For this review, take the finished solid that the model builds, in its own axes (mm). Face numbers are marked on the shaded views. A direction names the side the tool comes from. Coordinates: 2 decimals unless noted, no trailing zeros. Order: outer loops, then holes, each group sorted by start corner. A loop starts at its lowest first (then second) coordinate and runs counter-clockwise, first axis right, second up. Notation, with made-up numbers: (3.25, 55) -> (47.25, 55) arc R35 cw to (47.25, 91) -> close; hole circle Ø5 at (-24.75, -2.5). An arc over 180 degrees is marked (long way). Answer as a JSON object with one key per item and string values. Group by question number.
1) Draft analysis for pull direction Y (two halves, no side actions). For the marked faces 4, 5, 6 and 7, state which applies: +Y half, -Y half, draft (parallel to the pull), parting line (faces both ways), or undercut.
2) Add section D-D, the plane x = 58.5. Write out the cut boundary in (y, z).
3) Add section A-A, the plane x = 108. Write out the cut boundary in (y, z), then the cut area to 4 significant figures.
4) Machinability: for the marked faces 1, 2 and 3, which of the approach directions +Z, -Z, +X, -X, +Y, -Y give a long, thin tool a straight path to every point of the face, cutting with its end or side? Answer none if there is none.
5) Add section C-C, the plane x = 14. Write out the cut boundary in (y, z).
6) Add section B-B, the plane y = 26. Write out the cut boundary in (x, z).
7) For pin 1 (10 mm diameter, centred on x = 111.5, y = 15.5, fed in from -Z); pin 2 (11 mm diameter, centred on y = 26, z = 9.75, fed in from -X); pin 3 (5 mm diameter, centred on x = 62, y = 31.5, fed in from -Z); pin 4 (6 mm diameter, centred on y = 25.5, z = 11.5, fed in from +X), all flat-tipped, find the tip position at first contact; note any pin that passes through.
8) Wall thickness on L1, parallel to Y at x = 55, z = 13.25; L2, parallel to Z at x = 127, y = 26; L3, parallel to Y at x = 12, z = 9.75: over which ranges is each line inside the solid? List them lowest first.
from build123d import *

# Parameters (mm, degrees)
BOSS_EXTRUDE1_DEPTH = 19.5
SKETCH2_R           = 8.5
CUT_EXTRUDE2_DEPTH  = 7
SKETCH3_R           = 4.5
CUT_EXTRUDE3_DEPTH  = 142.000886522
SKETCH5_R           = 6
CUT_EXTRUDE4_DEPTH  = 10
CUT_EXTRUDE5_START  = -10
SKETCH6_R           = 6
CUT_EXTRUDE5_DEPTH  = 10


with BuildPart() as part:
    # Model → Boss-Extrude1 (new body)
    with BuildSketch(Plane.XY):
        Polygon((0, 41), (0, 10), (10, 0), (120, 0), (130, 10), (130, 41), (120, 51), (10, 51), align=None)
        with BuildLine():
            Line((24.5, 15), (105.5, 15))
            ThreePointArc((105.5, 15), (110.096194078, 16.903805922), (112, 21.5))
            Line((112, 21.5), (112, 29.5))
            ThreePointArc((112, 29.5), (110.096194078, 34.096194078), (105.5, 36))
            Line((105.5, 36), (24.5, 36))
            ThreePointArc((24.5, 36), (19.903805922, 34.096194078), (18, 29.5))
            Line((18, 29.5), (18, 21.5))
            ThreePointArc((18, 21.5), (19.903805922, 16.903805922), (24.5, 15))
        make_face(mode=Mode.SUBTRACT)
    extrude(amount=BOSS_EXTRUDE1_DEPTH)

    # Sketch2 → Cut-Extrude2 (cut)
    with BuildSketch(Plane.ZY):
        with Locations((9.75, 26)):
            Circle(SKETCH2_R)
    extrude(amount=-CUT_EXTRUDE2_DEPTH, mode=Mode.SUBTRACT)

    # Sketch3 → Cut-Extrude3 (cut, through all)
    with BuildSketch(Plane.ZY):
        with Locations((9.75, 26)):
            Circle(SKETCH3_R)
    extrude(amount=-CUT_EXTRUDE3_DEPTH, mode=Mode.SUBTRACT)

    # Sketch5 → Cut-Extrude4 (cut)
    with BuildSketch(Plane.ZY.offset(-7)):
        with Locations((9.75, 26)):
            Circle(SKETCH5_R)
    extrude(amount=-CUT_EXTRUDE4_DEPTH, mode=Mode.SUBTRACT)

    # Sketch6 → Cut-Extrude5 (cut)
    with BuildSketch(Plane(origin=(130, 0, 0), x_dir=(0, 0, -1), z_dir=(1, 0, 0)).offset(CUT_EXTRUDE5_START)):
        with Locations(Location((-9.75, 26, 0), (0, 0, 180))):
            Circle(SKETCH6_R)
    extrude(amount=CUT_EXTRUDE5_DEPTH, mode=Mode.SUBTRACT)


solid = part.part
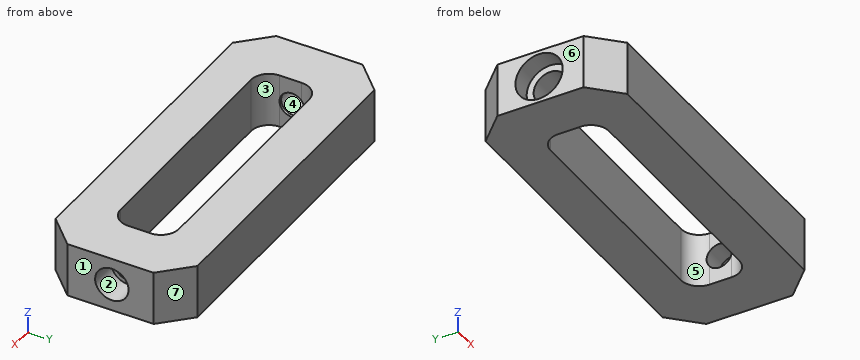
Output values:
{
 "1": {"face 4": "undercut", "face 5": "undercut", "face 6": "draft", "face 7": "+Y half"},
 "2": {"outline": "(0, 0) -> (15, 0) -> (15, 19.5) -> (0, 19.5) -> close; (36, 0) -> (51, 0) -> (51, 19.5) -> (36, 19.5) -> close"},
 "3": {"outline": "(0, 0) -> (15.5, 0) -> (15.5, 19.5) -> (0, 19.5) -> close; (35.5, 0) -> (51, 0) -> (51, 19.5) -> (35.5, 19.5) -> close", "area": "604.5 mm²"},
 "4": {"face 1": "+Z, -Z, +X, +Y, -Y", "face 2": "+X", "face 3": "+Z, -Z"},
 "5": {"outline": "(0, 0) -> (51, 0) -> (51, 19.5) -> (0, 19.5) -> close; hole circle Ø12 at (26, 9.75)"},
 "6": {"outline": "(0, 0) -> (18, 0) -> (18, 5.25) -> (17, 5.25) -> (17, 3.75) -> (7, 3.75) -> (7, 1.25) -> (0, 1.25) -> close; (0, 18.25) -> (7, 18.25) -> (7, 15.75) -> (17, 15.75) -> (17, 14.25) -> (18, 14.25) -> (18, 19.5) -> (0, 19.5) -> close; (112, 0) -> (130, 0) -> (130, 3.75) -> (120, 3.75) -> (120, 5.25) -> (112, 5.25) -> close; (112, 14.25) -> (120, 14.25) -> (120, 15.75) -> (130, 15.75) -> (130, 19.5) -> (112, 19.5) -> close"},
 "7": {"pin 1": "stops at z = 0", "pin 2": "stops at x = 17", "pin 3": "passes through", "pin 4": "stops at x = 120"},
 "8": {"L1": "y = 0 to 15, 36 to 51", "L2": "z = 0 to 3.75, 15.75 to 19.5", "L3": "y = 0 to 20, 32 to 51"}
}
